Input: dimensioned drawing with shaded views. Units: mm. Origin: part minimum x, y, z. Coordinates: 2 decimals unless noted, no trailing zeros. Order: outer loops, then holes, each group sorted by start corner. A loop starts at its lowest first (then second) coordinate and runs counter-clockwise, first axis right, second up. Notation, with made-up numbers: (13.25, 4.5) -> (21.25, 4.5) arc R20 cw to (21.25, 19.5) -> close; hole circle Ø4 at (39, -37). An arc over 180 degrees is marked (long way). Answer in a Markdown table with one row per item. Add a question column.
1) Section query A-A on z = 128.5. Return the cut outline in (x, y), then the cut area to 3 significant figures.
2) Contact query for a flat-ended pin moving along its axis: P1, Ø3, axis at y = 3, z = 103.5, coming from the -X side. Output: stop coordinate, or through.
3) Ray query, line 1 (X direction, y = 19.75, z = 128); line 2 (X direction, y = 23.25, z = 105). Return the intervals inside material, ascending. Write a range as from..to.
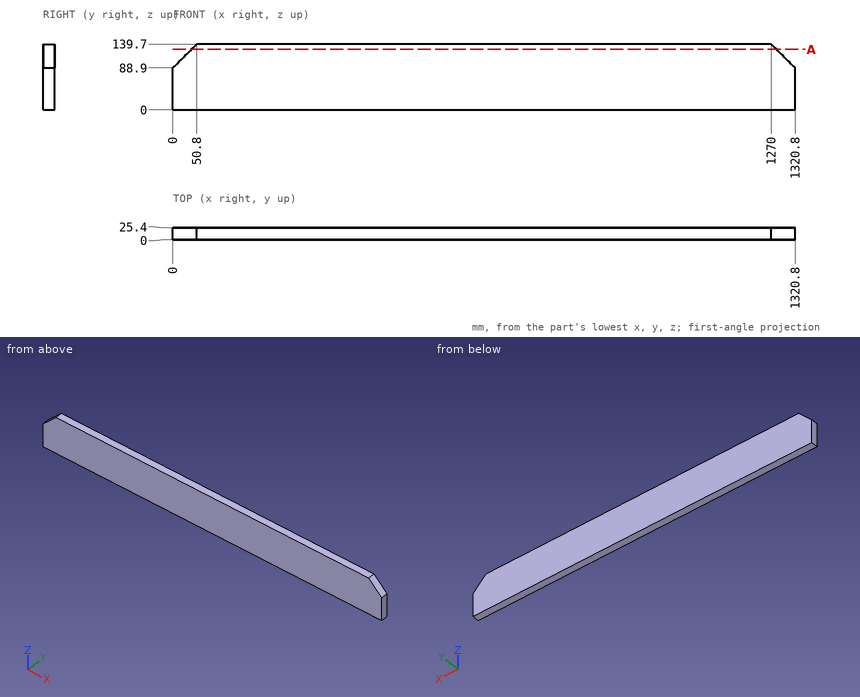
Result:
| question | item | result |
|---|---|---|
| 1 | outline | (39.6, 0) -> (1281.2, 0) -> (1281.2, 25.4) -> (39.6, 25.4) -> close |
| 1 | area | 31,500 mm2 |
| 2 | P1 | x = 13.1 |
| 3 | line 1 | 39.1..1281.7 |
| 3 | line 2 | 16.1..1304.7 |
